Can you work these out from the model? Positions are in its coordinate system, mm. Give positions to 0.01 mm unless a question says otherwise; leave off trailing zeros. One line per item, written item: value.
from build123d import *

# Parameters (mm, degrees)
SKETCH1_R           = 3.52998588
BOSS_EXTRUDE1_DEPTH = 362.74375


with BuildPart() as part:
    # Sketch1 → Boss-Extrude1 (new, symmetric)
    with BuildSketch(Plane.XY):
        with BuildLine():
            Line((14.49994, -4), (13.24247465, -4))
            ThreePointArc((13.24247465, -4), (12.88892126, -4.146446609), (12.74247465, -4.5))
            Line((12.74247465, -4.5), (12.74247465, -7.732519321))
            ThreePointArc((12.74247465, -7.732519321), (12.602449697, -8.097296796), (12.242781236, -8.249967))
            Line((12.242781236, -8.249967), (10.260188032, -8.249967))
            ThreePointArc((10.260188032, -8.249967), (10.068847082, -8.211906919), (9.906636056, -8.103520976))
            Line((9.906636056, -8.103520976), (5.981117769, -4.178002689))
            ThreePointArc((5.981117769, -4.178002689), (5.872731827, -4.015791664), (5.834671745, -3.824450713))
            Line((5.834671745, -3.824450713), (5.834671745, -1.01249595))
            Line((5.834671745, -1.01249595), (5.834671745, 0.88749645))
            Line((5.834671745, 0.88749645), (5.834671745, 3.824450713))
            ThreePointArc((5.834671745, 3.824450713), (5.872731827, 4.015791664), (5.981117769, 4.178002689))
            Line((5.981117769, 4.178002689), (9.906636056, 8.103520976))
            ThreePointArc((9.906636056, 8.103520976), (10.068847082, 8.211906919), (10.260188032, 8.249967))
            Line((10.260188032, 8.249967), (12.242781236, 8.249967))
            ThreePointArc((12.242781236, 8.249967), (12.602449697, 8.097296796), (12.74247465, 7.732519321))
            Line((12.74247465, 7.732519321), (12.74247465, 4.5))
            ThreePointArc((12.74247465, 4.5), (12.88892126, 4.146446609), (13.24247465, 4))
            Line((13.24247465, 4), (14.49994, 4))
            ThreePointArc((14.49994, 4), (14.853493391, 4.146446609), (14.99994, 4.5))
            Line((14.99994, 4.5), (14.99994, 12.999948))
            ThreePointArc((14.99994, 12.999948), (14.414155906, 14.414155906), (12.999948, 14.99994))
            Line((12.999948, 14.99994), (4.5, 14.99994))
            ThreePointArc((4.5, 14.99994), (4.146446609, 14.853493391), (4, 14.49994))
            Line((4, 14.49994), (4, 13.24247465))
            ThreePointArc((4, 13.24247465), (4.146446609, 12.88892126), (4.5, 12.74247465))
            Line((4.5, 12.74247465), (7.732519321, 12.74247465))
            ThreePointArc((7.732519321, 12.74247465), (8.097296796, 12.602449697), (8.249967, 12.242781236))
            Line((8.249967, 12.242781236), (8.249967, 10.260188032))
            ThreePointArc((8.249967, 10.260188032), (8.211906919, 10.068847082), (8.103520976, 9.906636056))
            Line((8.103520976, 9.906636056), (4.178002689, 5.981117769))
            ThreePointArc((4.178002689, 5.981117769), (4.015791664, 5.872731827), (3.824450713, 5.834671745))
            Line((3.824450713, 5.834671745), (0.9499962, 5.834671745))
            Line((0.9499962, 5.834671745), (-0.9499962, 5.834671745))
            Line((-0.9499962, 5.834671745), (-3.824450713, 5.834671745))
            ThreePointArc((-3.824450713, 5.834671745), (-4.015791664, 5.872731827), (-4.178002689, 5.981117769))
            Line((-4.178002689, 5.981117769), (-8.103520976, 9.906636056))
            ThreePointArc((-8.103520976, 9.906636056), (-8.211906919, 10.068847082), (-8.249967, 10.260188032))
            Line((-8.249967, 10.260188032), (-8.249967, 12.242781236))
            ThreePointArc((-8.249967, 12.242781236), (-8.097296796, 12.602449697), (-7.732519321, 12.74247465))
            Line((-7.732519321, 12.74247465), (-4.5, 12.74247465))
            ThreePointArc((-4.5, 12.74247465), (-4.146446609, 12.88892126), (-4, 13.24247465))
            Line((-4, 13.24247465), (-4, 14.49994))
            ThreePointArc((-4, 14.49994), (-4.146446609, 14.853493391), (-4.5, 14.99994))
            Line((-4.5, 14.99994), (-12.999948, 14.99994))
            ThreePointArc((-12.999948, 14.99994), (-14.414155906, 14.414155906), (-14.99994, 12.999948))
            Line((-14.99994, 12.999948), (-14.99994, 4.5))
            ThreePointArc((-14.99994, 4.5), (-14.853493391, 4.146446609), (-14.49994, 4))
            Line((-14.49994, 4), (-13.24247465, 4))
            ThreePointArc((-13.24247465, 4), (-12.88892126, 4.146446609), (-12.74247465, 4.5))
            Line((-12.74247465, 4.5), (-12.74247465, 7.732519321))
            ThreePointArc((-12.74247465, 7.732519321), (-12.602449697, 8.097296796), (-12.242781236, 8.249967))
            Line((-12.242781236, 8.249967), (-10.260188032, 8.249967))
            ThreePointArc((-10.260188032, 8.249967), (-10.068847082, 8.211906919), (-9.906636056, 8.103520976))
            Line((-9.906636056, 8.103520976), (-5.981117769, 4.178002689))
            ThreePointArc((-5.981117769, 4.178002689), (-5.872731827, 4.015791664), (-5.834671745, 3.824450713))
            Line((-5.834671745, 3.824450713), (-5.834671745, 0.88749645))
            Line((-5.834671745, 0.88749645), (-5.834671745, -1.01249595))
            Line((-5.834671745, -1.01249595), (-5.834671745, -3.824450713))
            ThreePointArc((-5.834671745, -3.824450713), (-5.872731827, -4.015791664), (-5.981117769, -4.178002689))
            Line((-5.981117769, -4.178002689), (-9.906636056, -8.103520976))
            ThreePointArc((-9.906636056, -8.103520976), (-10.068847082, -8.211906919), (-10.260188032, -8.249967))
            Line((-10.260188032, -8.249967), (-12.242781236, -8.249967))
            ThreePointArc((-12.242781236, -8.249967), (-12.602449697, -8.097296796), (-12.74247465, -7.732519321))
            Line((-12.74247465, -7.732519321), (-12.74247465, -4.5))
            ThreePointArc((-12.74247465, -4.5), (-12.88892126, -4.146446609), (-13.24247465, -4))
            Line((-13.24247465, -4), (-14.49994, -4))
            ThreePointArc((-14.49994, -4), (-14.853493391, -4.146446609), (-14.99994, -4.5))
            Line((-14.99994, -4.5), (-14.99994, -12.999948))
            ThreePointArc((-14.99994, -12.999948), (-14.414155906, -14.414155906), (-12.999948, -14.99994))
            Line((-12.999948, -14.99994), (-4.5, -14.99994))
            ThreePointArc((-4.5, -14.99994), (-4.146446609, -14.853493391), (-4, -14.49994))
            Line((-4, -14.49994), (-4, -13.24247465))
            ThreePointArc((-4, -13.24247465), (-4.146446609, -12.88892126), (-4.5, -12.74247465))
            Line((-4.5, -12.74247465), (-7.732519321, -12.74247465))
            ThreePointArc((-7.732519321, -12.74247465), (-8.097296796, -12.602449697), (-8.249967, -12.242781236))
            Line((-8.249967, -12.242781236), (-8.249967, -10.260188032))
            ThreePointArc((-8.249967, -10.260188032), (-8.211906919, -10.068847082), (-8.103520976, -9.906636056))
            Line((-8.103520976, -9.906636056), (-4.178002689, -5.981117769))
            ThreePointArc((-4.178002689, -5.981117769), (-4.015791664, -5.872731827), (-3.824450713, -5.834671745))
            Line((-3.824450713, -5.834671745), (-0.9499962, -5.834671745))
            Line((-0.9499962, -5.834671745), (0.9499962, -5.834671745))
            Line((0.9499962, -5.834671745), (3.824450713, -5.834671745))
            ThreePointArc((3.824450713, -5.834671745), (4.015791664, -5.872731827), (4.178002689, -5.981117769))
            Line((4.178002689, -5.981117769), (8.103520976, -9.906636056))
            ThreePointArc((8.103520976, -9.906636056), (8.211906919, -10.068847082), (8.249967, -10.260188032))
            Line((8.249967, -10.260188032), (8.249967, -12.242781236))
            ThreePointArc((8.249967, -12.242781236), (8.097296796, -12.602449697), (7.732519321, -12.74247465))
            Line((7.732519321, -12.74247465), (4.5, -12.74247465))
            ThreePointArc((4.5, -12.74247465), (4.146446609, -12.88892126), (4, -13.24247465))
            Line((4, -13.24247465), (4, -14.49994))
            ThreePointArc((4, -14.49994), (4.146446609, -14.853493391), (4.5, -14.99994))
            Line((4.5, -14.99994), (12.999948, -14.99994))
            ThreePointArc((12.999948, -14.99994), (14.414155906, -14.414155906), (14.99994, -12.999948))
            Line((14.99994, -12.999948), (14.99994, -4.5))
            ThreePointArc((14.99994, -4.5), (14.853493391, -4.146446609), (14.49994, -4))
        make_face()
        Circle(SKETCH1_R, mode=Mode.SUBTRACT)
        with BuildLine():
            Line((-12.6999492, -13.6999452), (-9.880960476, -13.6999452))
            ThreePointArc((-9.880960476, -13.6999452), (-9.61155387, -13.58835333), (-9.499962, -13.318946724))
            Line((-9.499962, -13.318946724), (-9.499962, -9.87996048))
            ThreePointArc((-9.499962, -9.87996048), (-9.611260978, -9.611260978), (-9.87996048, -9.499962))
            Line((-9.87996048, -9.499962), (-13.318946724, -9.499962))
            ThreePointArc((-13.318946724, -9.499962), (-13.58835333, -9.61155387), (-13.6999452, -9.880960476))
            Line((-13.6999452, -9.880960476), (-13.6999452, -12.6999492))
            ThreePointArc((-13.6999452, -12.6999492), (-13.407053153, -13.407053153), (-12.6999492, -13.6999452))
        make_face(mode=Mode.SUBTRACT)
        with BuildLine():
            Line((13.6999452, -12.6999492), (13.6999452, -9.880960476))
            ThreePointArc((13.6999452, -9.880960476), (13.58835333, -9.61155387), (13.318946724, -9.499962))
            Line((13.318946724, -9.499962), (9.87996048, -9.499962))
            ThreePointArc((9.87996048, -9.499962), (9.611260978, -9.611260978), (9.499962, -9.87996048))
            Line((9.499962, -9.87996048), (9.499962, -13.318946724))
            ThreePointArc((9.499962, -13.318946724), (9.61155387, -13.58835333), (9.880960476, -13.6999452))
            Line((9.880960476, -13.6999452), (12.6999492, -13.6999452))
            ThreePointArc((12.6999492, -13.6999452), (13.407053153, -13.407053153), (13.6999452, -12.6999492))
        make_face(mode=Mode.SUBTRACT)
        with BuildLine():
            Line((9.87996048, 9.499962), (13.318946724, 9.499962))
            ThreePointArc((13.318946724, 9.499962), (13.58835333, 9.61155387), (13.6999452, 9.880960476))
            Line((13.6999452, 9.880960476), (13.6999452, 12.6999492))
            ThreePointArc((13.6999452, 12.6999492), (13.407053153, 13.407053153), (12.6999492, 13.6999452))
            Line((12.6999492, 13.6999452), (9.880960476, 13.6999452))
            ThreePointArc((9.880960476, 13.6999452), (9.61155387, 13.58835333), (9.499962, 13.318946724))
            Line((9.499962, 13.318946724), (9.499962, 9.87996048))
            ThreePointArc((9.499962, 9.87996048), (9.611260978, 9.611260978), (9.87996048, 9.499962))
        make_face(mode=Mode.SUBTRACT)
        with BuildLine():
            Line((-13.6999452, 12.6999492), (-13.6999452, 9.880960476))
            ThreePointArc((-13.6999452, 9.880960476), (-13.58835333, 9.61155387), (-13.318946724, 9.499962))
            Line((-13.318946724, 9.499962), (-9.87996048, 9.499962))
            ThreePointArc((-9.87996048, 9.499962), (-9.611260978, 9.611260978), (-9.499962, 9.87996048))
            Line((-9.499962, 9.87996048), (-9.499962, 13.318946724))
            ThreePointArc((-9.499962, 13.318946724), (-9.61155387, 13.58835333), (-9.880960476, 13.6999452))
            Line((-9.880960476, 13.6999452), (-12.6999492, 13.6999452))
            ThreePointArc((-12.6999492, 13.6999452), (-13.407053153, 13.407053153), (-13.6999452, 12.6999492))
        make_face(mode=Mode.SUBTRACT)
    extrude(amount=BOSS_EXTRUDE1_DEPTH, both=True)


solid = part.part
1) I need wall thicknesses on L1, parallel to Y at x = 13.5, z = -34; L2, parallel to X at y = -10.75, z = -164. Which ranges of each line are inside material? Lowest first, please.
Answer list:
L1: y = -14.94 to -13.3, -9.55 to -4, 4 to 9.55, 13.3 to 14.94
L2: x = -15 to -13.7, -9.5 to -8.25, 8.25 to 9.5, 13.7 to 15
2) Will these pins go through, and if not, where does the flat tip stop? pin 1 (1.4 mm diameter, centred on x = 14, z = -13, fed in from -Y); pin 2 (1.4 mm diameter, centred on y = 14, z = 144, fed in from -X); pin 3 (6 mm diameter, centred on x = 0, z = -257.5, fed in from -Y).
Answer list:
pin 1: stops at y = -14.98
pin 2: stops at x = -14.98
pin 3: stops at y = -5.83
3) If we section it at A-A (z = -84.5): State how many separate pieces and enclosed holes the cut face has, and give its area (3 significant figures).
Answer list:
separate pieces: 1
enclosed holes: 5
area: 331 mm^2
